from build123d import *

# Parameters (mm, degrees)
SKETCH1_R           = 35.15
SKETCH1_R_2         = 1.75
BOSS_EXTRUDE2_DEPTH = 3
SKETCH3_R           = 27.5
SKETCH3_R_2         = 25.5
BOSS_EXTRUDE3_DEPTH = 28.7


with BuildPart() as part:
    # Sketch1 → Boss-Extrude2 (new body)
    with BuildSketch(Plane.XY):
        Circle(SKETCH1_R)
        with Locations((0, 31.5)):
            Circle(SKETCH1_R_2, mode=Mode.SUBTRACT)
        with Locations((22.273863607, 22.273863607)):
            Circle(SKETCH1_R_2, mode=Mode.SUBTRACT)
        with Locations((31.5, 0)):
            Circle(SKETCH1_R_2, mode=Mode.SUBTRACT)
        with Locations((22.273863607, -22.273863607)):
            Circle(SKETCH1_R_2, mode=Mode.SUBTRACT)
        with Locations((0, -31.5)):
            Circle(SKETCH1_R_2, mode=Mode.SUBTRACT)
        with Locations((-22.273863607, -22.273863607)):
            Circle(SKETCH1_R_2, mode=Mode.SUBTRACT)
        with Locations((-31.5, 0)):
            Circle(SKETCH1_R_2, mode=Mode.SUBTRACT)
        with Locations((-22.273863607, 22.273863607)):
            Circle(SKETCH1_R_2, mode=Mode.SUBTRACT)
    extrude(amount=BOSS_EXTRUDE2_DEPTH)

    # Sketch3 → Boss-Extrude3 (add)
    with BuildSketch(Plane.XY.offset(3)):
        Circle(SKETCH3_R)
        Circle(SKETCH3_R_2, mode=Mode.SUBTRACT)
    extrude(amount=BOSS_EXTRUDE3_DEPTH)


solid = part.part
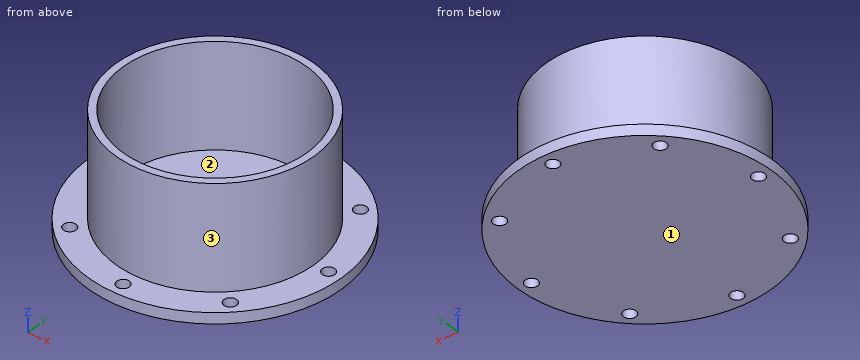
Work out the finished part from the listing and answer in its coordinate system (mm). Face numbers are marked on the shaded views. Give positions to 0.01 mm unless a question says otherwise; leave off trailing zeros. Order: outer loops, then holes, each group sorted by start corner. A loop starts at its lowest first (then second) coordinate and runs counter-clockwise, first axis right, second up. Notation, with made-up numbers: (56, -36) -> (61, -36) arc R22 ccw to (61, 2) -> close; hole circle Ø5 at (58, 7.5). An arc over 180 degrees is marked (long way). Answer as a JSON object with one key per item and string values. Group by question number.
1. Consider line 1 along Y through (x, z) = (0, 1); line 2 along Z through (x, y) = (-11, 31); line 3 along X through (y, z) = (-19, 13.5). Determine where each line is inside the solid, lowest interval first. Write a range as [from, to].
2. Flat-ended cylindrical pins translate along their axes: pin 1 Ø4 at (x, y) = (0, 31.5) entering from +Z; pin 2 Ø10 at (x, z) = (14.5, 13) entering from +Y; pin 3 Ø12 at (y, z) = (13.5, 28) entering from -X. Find the tip coordinate at first contact, or state that the pin passes through.
3. Section C-C on y = -31.5 is taken. Determine the outline of the cut face in (x, z).
4. The mould has two halves that part along X. Classify the marked faces 1, 2 and 3: released by +X, released by -X, zero draft, split by the parting line, or undercut.
5. Section D-D on z = 26.5 is taken. Determine the outline of the cut face in (x, y).
6. Section A-A on y = 0 is taken. Determine the outline of the cut face in (x, z), plus the area to 3 significant figures.
Result sheet:
{
 "1": {"line 1": "y = [-35.15, -33.25], [-29.75, 29.75], [33.25, 35.15]", "line 2": "z = [0, 3]", "line 3": "x = [-19.88, -17.01], [17.01, 19.88]"},
 "2": {"pin 1": "stops at z = 3", "pin 2": "stops at y = 25.81", "pin 3": "stops at x = -26.46"},
 "3": {"outline": "(-15.6, 0) -> (-1.75, 0) -> (-1.75, 3) -> (-15.6, 3) -> close; (1.75, 0) -> (15.6, 0) -> (15.6, 3) -> (1.75, 3) -> close"},
 "4": {"face 1": "zero draft", "face 2": "undercut", "face 3": "split by the parting line"},
 "5": {"outline": "circle Ø55 at (0, 0); hole circle Ø51 at (0, 0)"},
 "6": {"outline": "(-35.15, 0) -> (-33.25, 0) -> (-33.25, 3) -> (-35.15, 3) -> close; (-29.75, 0) -> (29.75, 0) -> (29.75, 3) -> (27.5, 3) -> (27.5, 31.7) -> (25.5, 31.7) -> (25.5, 3) -> (-25.5, 3) -> (-25.5, 31.7) -> (-27.5, 31.7) -> (-27.5, 3) -> (-29.75, 3) -> close; (33.25, 0) -> (35.15, 0) -> (35.15, 3) -> (33.25, 3) -> close", "area": "305 mm^2"}
}
